Geometry: final body of the model. Coordinates: model frame, mm. Face numbers are marked on the shaded views. A direction names the side the tool comes from. Give positions to 0.01 mm unless a question says otherwise; leave off trailing zeros. Write each loop counter-clockwise with the first axis right and the second up, starting at its lowest first coordinate (ties: lowest second). Pieces come first, ordered by that corner, then holes. Notation, with made-up numbers: M 4,-31.5 L 34,-31.5 A9 ccw 34,-24.5 Z; hole C 82,25 d10. An arc over 180 degrees is marked long. Answer as a JSON object with one key per item and string values.
from build123d import *

# Parameters (mm, degrees)
F1_DEPTH = 10
F2_R     = 10.061919
F3_DEPTH = 3
F4_R     = 2.15
F5_DEPTH = 25
F6_R     = 0.5


with BuildPart() as f1:
    # F0 (on Top) → F1 (new body)
    with BuildSketch(Plane.XY):
        Polygon((6.580053, 3.844854), (-0.039715, 7.62092), (-6.619768, 3.776066), (-6.580053, -3.844854), (0.039715, -7.62092), (6.619768, -3.776066), align=None)
    extrude(amount=F1_DEPTH)

    # F2 (on face) → F3 (join)
    with BuildSketch(Plane.XY.offset(10)):
        Circle(F2_R)
    extrude(amount=F3_DEPTH)

    # F4 (on face) → F5 (cut)
    with BuildSketch(Plane.XY.offset(13)):
        Circle(F4_R)
    extrude(amount=-F5_DEPTH, mode=Mode.SUBTRACT)

    # F6
    f6_edges = [f1.edges().sort_by_distance(p)[0] for p in [
        (-0.039715, 7.62092, 5),
        (6.580053, 3.844854, 5),
        (6.619768, -3.776066, 5),
        (0.039715, -7.62092, 5),
        (-6.580053, -3.844854, 5),
        (-6.619768, 3.776066, 5),
        (-3.329741, 5.698493, 0),
        (-6.59991, -0.034394, 0),
        (-3.270169, -5.732887, 0),
        (3.329741, -5.698493, 0),
        (6.59991, 0.034394, 0),
        (3.270169, 5.732887, 0),
        (-2.15, 0, 0),
    ]]
    fillet(f6_edges, radius=F6_R)


solid = f1.part
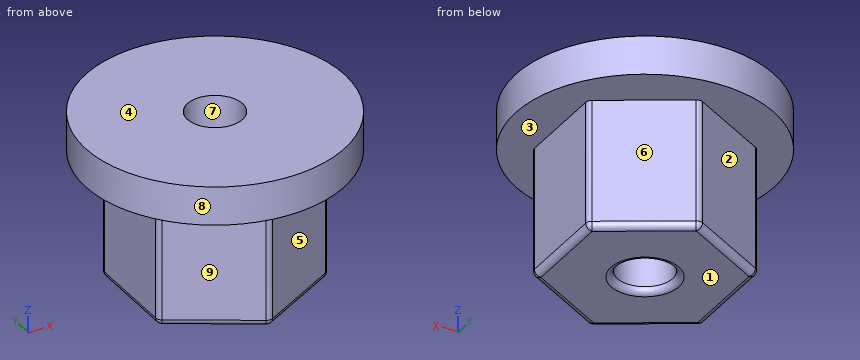
1) Line query: line 1 (Y direction, x = 0, z = 7.5); line 2 (Z direction, x = 4, y = -5.25); line 3 (Z direction, x = -5.75, y = 5.5). Output: solid intervals per line, ascending. Write a range as from..to.
Geometry check:
{"line 1": "y = -7.54..-2.15, 2.15..7.54", "line 2": "z = 0.28..13", "line 3": "z = 10..13"}
2) Contact query for flat-ended pins moving along their axis: P1, Ø4, axis at x = 1, z = 5.5, coming from the -Y side; P2, Ø5, axis at x = 0, y = 0, coming from the -Z side; P3, Ø1.5, axis at x = -3, z = 3, coming from the -Y side. Output: stop coordinate, or through.
Geometry check:
{"P1": "stops at y = -7.54", "P2": "stops at z = 0.02", "P3": "stops at y = -6.31"}
3) Cut plane B-B on x = -8.5. Return loops of the section in (y, z).
Geometry check:
{"outline": "M -5.38,10 L 5.38,10 L 5.38,13 L -5.38,13 Z"}
4) Pull-direction query (Y, two-part tool) for the marked faces 6, 7, 8 and 9; classes: pulls with the +Y half, pulls with the -Y half, needs draft (parallel to the pull), parting line crosses it, or undercut.
Geometry check:
{"face 6": "pulls with the +Y half", "face 7": "undercut", "face 8": "parting line crosses it", "face 9": "pulls with the -Y half"}
5) Set-up query: the marked faces 1, 2, 3, 4 and 5. Return all of +Z, -Z, +X, -X, +Y, -Y with unobstructed straight access to the full face (end or side cutting, diameter ignored); none if empty.
Geometry check:
{"face 1": "-Z, +X, -X, +Y, -Y", "face 2": "-Z, -X, +Y", "face 3": "-Z", "face 4": "+Z, +X, -X, +Y, -Y", "face 5": "-Z, +X, -Y"}
6) Cut plane C-C on x = 8. Return loops of the section in (y, z), and give its area (3 significant figures).
Geometry check:
{"outline": "M -6.1,10 L 6.1,10 L 6.1,13 L -6.1,13 Z", "area": "36.6 mm2"}
7) Cut plane A-A on z = 3. Return loops of the section in (x, y), and give its area (3 significant figures).
Geometry check:
{"outline": "M -6.62,3.49 L -6.58,-3.56 A0.5 ccw -6.33,-3.99 L -0.21,-7.48 A0.5 ccw 0.29,-7.48 L 6.37,-3.92 A0.5 ccw 6.62,-3.49 L 6.58,3.56 A0.5 ccw 6.33,3.99 L 0.21,7.48 A0.5 ccw -0.29,7.48 L -6.37,3.92 A0.5 ccw Z; hole C 0,0 d4.3", "area": "136 mm2"}
